from build123d import *

# Parameters (mm, degrees)
SKETCH_1_R      = 2.5
SKETCH_1_R_2    = 1.410646597
EXTRUDE_1_DEPTH = 3
SKETCH_2_R      = 3
EXTRUDE_2_DEPTH = 16.5
EXTRUDE_START   = 15
SKETCH_3_R      = 2.5
EXTRUDE_3_DEPTH = 15


with BuildPart() as part:
    # Эскиз1 → Бобышка-Вытянуть1 (new body)
    with BuildSketch(Plane.XY):
        with Locations((0.280254447, 0.00265159)):
            Circle(SKETCH_1_R)
        with Locations((0.280254447, 0.00265159)):
            Circle(SKETCH_1_R_2, mode=Mode.SUBTRACT)
    extrude(amount=-EXTRUDE_1_DEPTH)

    # Эскиз2 → Бобышка-Вытянуть2 (add)
    with BuildSketch(Plane.XY):
        with Locations(Location((0.280254447, 0.00265159, 0), (0, 0, 180))):
            Circle(SKETCH_2_R)
    extrude(amount=EXTRUDE_2_DEPTH)

    # Эскиз3 → Бобышка-Вытянуть3 (add)
    with BuildSketch(Plane.XY.offset(16.5).offset(EXTRUDE_START)):
        with Locations((0.280254447, 0.00265159)):
            Circle(SKETCH_3_R)
    extrude(amount=-EXTRUDE_3_DEPTH)


solid = part.part
The listing builds one solid part. Answer for the finished solid, in the listing's coordinates (mm). A direction names the side the tool comes from. Give positions to 0.01 mm unless a question says otherwise; leave off trailing zeros. Order: outer loops, then holes, each group sorted by start corner. A loop starts at its lowest first (then second) coordinate and runs counter-clockwise, first axis right, second up. Notation, with made-up numbers: (-16.75, 11.25) - (-12.75, 11.25) arc R16 cw to (-12.75, 40.25) - close; hole circle Ø6 at (36, 64.5). An arc over 180 degrees is marked (long way). Answer as CSV lines item,"result".
Q1. Determine the mould class of faces 3 (the face through (-0.26, -2.44, 24.1)), 4 (the face through (1.626, 0.426, -1.479)), 5 (the face through (0, 0, 31.5)), 6 (the face through (0, 0, 0)) for opening direction X: pulls with the +X half, pulls with the -X half, needs draft (parallel to the pull), parting line crosses it, or undercut.
Answer key:
face 3,"parting line crosses it"
face 4,"undercut"
face 5,"needs draft"
face 6,"undercut"
Q2. A cutting plane is placed at A-A, the plane x = 1.2. Determine the outline of the cut face in (y, z), and give its area (3 significant figures).
Answer key:
outline,"(-2.85, 0) - (-2.32, 0) - (-2.32, -3) - (-1.07, -3) - (-1.07, 0) - (1.07, 0) - (1.07, -3) - (2.33, -3) - (2.33, 0) - (2.86, 0) - (2.86, 16.5) - (2.33, 16.5) - (2.33, 31.5) - (-2.32, 31.5) - (-2.32, 16.5) - (-2.85, 16.5) - close"
area,"172 mm^2"
Q3. A cutting plane is placed at B-B, the plane y = 0.6. Determine the outline of the cut face in (x, z), and give its area (3 significant figures).
Answer key:
outline,"(-2.66, 0) - (-2.15, 0) - (-2.15, -3) - (-1, -3) - (-1, 0) - (1.56, 0) - (1.56, -3) - (2.71, -3) - (2.71, 0) - (3.22, 0) - (3.22, 16.5) - (2.71, 16.5) - (2.71, 31.5) - (-2.15, 31.5) - (-2.15, 16.5) - (-2.66, 16.5) - close"
area,"177 mm^2"
Q4. Straight lines are drawn through the part: L1, parallel to Z at x = -1.95, y = 1.8; L2, parallel to Z at x = -0.6, y = 1.05; L3, parallel to Y at x = 2.25, z = 4. For each, find the intervals that lie inside material, in ascending order.
Answer key:
L1,"z = 0 to 16.5"
L2,"z = 0 to 31.5"
L3,"y = -2.26 to 2.27"
Q5. Which of the six approach directions +Z, -Z, +X, -X, +Y, -Y give full straight-line access (tool end or side, diameter ignored) to faces 1 (the face through (-0.26, -2.44, -1.48)), 2 (the face through (3.277, -0.129, 8.134))?
Answer key:
face 1,"-Z"
face 2,"+Z, -Z"
Q6. A cutting plane is placed at D-D, the plane y = -1.8. Determine the outline of the cut face in (x, z).
Answer key:
outline,"(-2.12, 0) - (-1.45, 0) - (-1.45, -3) - (2.01, -3) - (2.01, 0) - (2.68, 0) - (2.68, 16.5) - (2.01, 16.5) - (2.01, 31.5) - (-1.45, 31.5) - (-1.45, 16.5) - (-2.12, 16.5) - close"
Q7. Each of these flat-tipped pins is pushed along its axis until it touches: pin 1 Ø2 at (x, z) = (-1, 20) entering from +Y; pin 2 Ø3 at (y, z) = (1, 20) entering from +X. Where does it stop, or does it pass through?
Answer key:
pin 1,"stops at y = 2.49"
pin 2,"stops at x = 2.78"
Q8. A cutting plane is placed at C-C, the plane z = 20.5. Determine the outline of the cut face in (x, y), and give its area (3 significant figures).
Answer key:
outline,"circle Ø5 at (0.28, 0)"
area,"19.6 mm^2"
